```python
from build123d import *

# Parameters (mm, degrees)
ESQUISSE1_W             = 180.475
ESQUISSE1_H             = 100
ESQUISSE1_R             = 5
BOSS_EXTRU_1_DEPTH      = 5
ESQUISSE2_W             = 8
ESQUISSE2_H             = 100
ENL_V_MAT_EXTRU_1_DEPTH = 5
ESQUISSE3_R             = 3
ENL_V_MAT_EXTRU_2_DEPTH = 5


with BuildPart() as part:
    # Esquisse1 → Boss.-Extru.1 (new body)
    with BuildSketch(Plane(origin=(0, 0, 0), x_dir=(1, 0, 0), z_dir=(0, 1, 0))):
        Rectangle(ESQUISSE1_W, ESQUISSE1_H)
        with Locations(Location((-72.19, 40, 0), (0, 0, 270))):
            Circle(ESQUISSE1_R, mode=Mode.SUBTRACT)
        with Locations(Location((72.19, 40, 0), (0, 0, 90))):
            Circle(ESQUISSE1_R, mode=Mode.SUBTRACT)
        with Locations(Location((72.19, -40, 0), (0, 0, 270))):
            Circle(ESQUISSE1_R, mode=Mode.SUBTRACT)
        with Locations(Location((-72.19, -40, 0), (0, 0, 90))):
            Circle(ESQUISSE1_R, mode=Mode.SUBTRACT)
        with Locations(Location((0, 0, 0), (0, 0, 270))):
            Circle(ESQUISSE1_R, mode=Mode.SUBTRACT)
    extrude(amount=BOSS_EXTRU_1_DEPTH)

    # Esquisse2 → Enlèv. mat.-Extru.1 (cut)
    with BuildSketch(Plane(origin=(0, 5, 0), x_dir=(1, 0, 0), z_dir=(0, 1, 0))):
        with Locations((-86.2375, 0)):
            Rectangle(ESQUISSE2_W, ESQUISSE2_H)
        with Locations((86.2375, 0)):
            Rectangle(ESQUISSE2_W, ESQUISSE2_H)
    extrude(amount=-ENL_V_MAT_EXTRU_1_DEPTH, mode=Mode.SUBTRACT)

    # Esquisse3 → Enlèv. mat.-Extru.2 (cut)
    with BuildSketch(Plane(origin=(0, 5, 0), x_dir=(1, 0, 0), z_dir=(0, 1, 0))):
        with Locations(Location((-30.8390625, 43.75, 0), (0, 0, 270))):
            Circle(ESQUISSE3_R)
        with Locations(Location((30.8390625, 43.75, 0), (0, 0, 270))):
            Circle(ESQUISSE3_R)
        with Locations(Location((30.8390625, -43.75, 0), (0, 0, 270))):
            Circle(ESQUISSE3_R)
        with Locations(Location((-30.8390625, -43.75, 0), (0, 0, 270))):
            Circle(ESQUISSE3_R)
    extrude(amount=-ENL_V_MAT_EXTRU_2_DEPTH, mode=Mode.SUBTRACT)


solid = part.part
```
Geometry: final body of the model. Coordinates: model frame, mm. Coordinates: 2 decimals unless noted, no trailing zeros. Order: outer loops, then holes, each group sorted by start corner. A loop starts at its lowest first (then second) coordinate and runs counter-clockwise, first axis right, second up. Notation, with made-up numbers: (6.5, 62) -> (58.5, 62) arc R25 cw to (58.5, 79) -> close; hole circle Ø10 at (-34, 61). An arc over 180 degrees is marked (long way). Write each question's results on one line, items separated by ' | '. Start each with the question number.
1) Cut plane B-B, the plane x = -72.19. Output: boundary loops of the cut face in (y, z), and give its area (3 significant figures).
2) Material intervals for line 1 along Z through (x, y) = (31, 0.3); line 2 along X through (y, z) = (1.2, -40); line 3 along Z through (x, y) = (71, 0.55), sorted ascending.
3) Cut plane D-D, the plane z = -38. Output: boundary loops of the cut face in (x, y).
4) Mould query, pull axis Z, two halves, no side actions, for faces 1 (the flat face through (-1, 2, 50)), 2 (the cylindrical face through (30.971, 2.535, 40.753)), 3 (the flat face through (-1, 2, -50)), 4 (the flat face through (82.238, 3, 1)). Classes: released by +Z, released by -Z, zero draft, split by the parting line, or undercut.
5) Cut plane C-C, the plane x = 0. Output: boundary loops of the cut face in (y, z).
6) Cut plane A-A, the plane z = 0. Output: boundary loops of the cut face in (x, y), and give its area (3 significant figures).
Checks:
1) outline: (0, -50) -> (5, -50) -> (5, -45) -> (0, -45) -> close; (0, -35) -> (5, -35) -> (5, 35) -> (0, 35) -> close; (0, 45) -> (5, 45) -> (5, 50) -> (0, 50) -> close | area: 400 mm^2
2) line 1: -50 to -46.75, -40.75 to 40.75, 46.75 to 50 | line 2: -82.24 to -77.19, -67.19 to 67.19, 77.19 to 82.24 | line 3: -50 to -44.86, -35.14 to 35.14, 44.86 to 50
3) outline: (-82.24, 0) -> (-76.77, 0) -> (-76.77, 5) -> (-82.24, 5) -> close; (-67.61, 0) -> (67.61, 0) -> (67.61, 5) -> (-67.61, 5) -> close; (76.77, 0) -> (82.24, 0) -> (82.24, 5) -> (76.77, 5) -> close
4) face 1: released by +Z | face 2: undercut | face 3: released by -Z | face 4: zero draft
5) outline: (0, -50) -> (5, -50) -> (5, -5) -> (0, -5) -> close; (0, 5) -> (5, 5) -> (5, 50) -> (0, 50) -> close
6) outline: (-82.24, 0) -> (-5, 0) -> (-5, 5) -> (-82.24, 5) -> close; (5, 0) -> (82.24, 0) -> (82.24, 5) -> (5, 5) -> close | area: 772 mm^2
